Autodesk Inventor part; units mm, degrees
ref_plane "YZ Plane" through (0, 0, 0) normal (1, 0, 0) x (0, 1, 0)
ref_plane "XZ Plane" through (0, 0, 0) normal (0, 1, 0) x (-1, 0, 0)
ref_plane "XY Plane" through (0, 0, 0) normal (0, 0, 1) x (1, 0, 0)
sketch "スケッチ1" plane through (0, 0, 0) normal (0, 0, 1) x (1, 0, 0)
  circle A0 centre (0, 0) radius 1.6
  circle A1 centre (0, 0) radius 5
  line L0 (-5, 0) -> (-5, 40)
  line L1 (-5, 40) -> (5, 40)
  line L2 (5, 40) -> (5, 0)
  dimension "d0" = 3.2
  dimension "d1" = 10
  dimension "d2" = 40
extrude "押し出し1" add sketch "スケッチ1" along normal blind 1.5
sketch "スケッチ2" plane through (0, 0, 1.5) normal (0, 0, 1) x (1, 0, 0)
  circle A0 centre (0, 0) radius 1.6
  circle A1 centre (0, 0) radius 3
  circle A2 centre (0, 4.5) radius 1.5
  circle A3 centre (0, 37) radius 1.5
  line L0 (5, 40) -> (-5, 40)
  line L1 (1.5, 37) -> (1.5, 4.5)
  line L2 (-1.5, 37) -> (-1.5, 4.5)
  dimension "d5" = 6
  dimension "d6" = 3
  dimension "d7" = 3
extrude "押し出し2" cut sketch "スケッチ2" against normal through all contours A2 | L2 A3 L1 A2 | A3
properties part number "kosinopich"
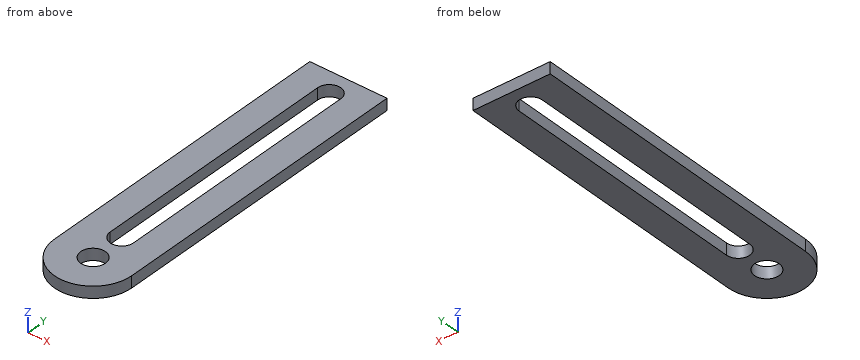
The model under review builds one solid part; all positions refer to its coordinate system, in mm. Coordinates: 2 decimals unless noted, no trailing zeros. Loops run counter-clockwise (first coordinate to the right, second up) from the corner with the lowest first, then second, coordinate; pieces in that order, holes last. Notation, with made-up numbers: M 38.5,64.25 L 74.5,64.25 A12 ccw 74.5,78.25 Z; hole C 2.5,35 d2. An arc over 180 degrees is marked long. Put each result on its own line as item: value. Start each with the question number.
Q1. Add section D-D (y = -1). Write out the cut boundary in (x, z), and give its area (3 significant figures).
Q2. Add section C-C (z = 1.1). Write out the cut boundary in (x, y), and give its area (3 significant figures).
Q3. Wall thickness on line 1 (X direction, y = 5, z = 0.65); line 2 (Y direction, x = -1, z = 1.3); line 3 (Y direction, x = 0, z = 0.9): over which ranges is each line inside the solid? List them lowest first.
Q4. Add section A-A (x = 0). Write out the cut boundary in (y, z), and give its area (3 significant figures).
Q5. Add section B-B (y = 25.5). Write out the cut boundary in (x, z).
Answers:
1. outline: M -4.9,0 L -1.25,0 L -1.25,1.5 L -4.9,1.5 Z; M 1.25,0 L 4.9,0 L 4.9,1.5 L 1.25,1.5 Z
1. area: 10.9 mm^2
2. outline: M -5,0 A5 ccw 5,0 L 5,40 L -5,40 Z; hole C 0,0 d3.2; hole M -1.5,4.5 A1.5 ccw 1.5,4.5 L 1.5,37 A1.5 ccw -1.5,37 Z
2. area: 327 mm^2
3. line 1: x = -5 to -1.5, 1.5 to 5
3. line 2: y = -4.9 to -1.25, 1.25 to 3.38, 38.12 to 40
3. line 3: y = -5 to -1.6, 1.6 to 3, 38.5 to 40
4. outline: M -5,0 L -1.6,0 L -1.6,1.5 L -5,1.5 Z; M 1.6,0 L 3,0 L 3,1.5 L 1.6,1.5 Z; M 38.5,0 L 40,0 L 40,1.5 L 38.5,1.5 Z
4. area: 9.45 mm^2
5. outline: M -5,0 L -1.5,0 L -1.5,1.5 L -5,1.5 Z; M 1.5,0 L 5,0 L 5,1.5 L 1.5,1.5 Z
